Design review of the part shown in the three views and the two pictorial views. Dimensions are in mm from the part's minimum x, y and z. A direction names the side the tool comes from. Give positions to 0.01 mm unless a question says otherwise; leave off trailing zeros. Loops run counter-clockwise (first coordinate to the right, second up) from the corner with the lowest first, then second, coordinate; pieces in that order, holes last. Notation, with made-up numbers: (20.5, -34) - (41.5, -34) arc R36 ccw to (41.5, 5) - close; hole circle Ø7 at (0.5, 81). An arc over 180 degrees is marked (long way). Use CSV: the item, a comma, the result in double quotes. Start each with the question number.
1. Wall thickness on line 1 (Y direction, x = 27, z = 18); line 2 (Y direction, x = 7, z = 19); line 3 (Z direction, x = 19.5, y = 10): over which ranges is each line inside the solid? List them lowest first.
2. For pin 1 (2 mm diameter, centred on y = 30.5, z = 16, fed in from +X); pin 2 (19 mm diameter, centred on x = 10, z = 15.5, fed in from -Y); pin 3 (3 mm diameter, centred on x = 19, y = 26.5, fed in from +Z), all flat-tipped, find the tip position at first contact; note any pin that passes through.
3. Take a section at D-D on z = 19. Give the boundary of the cut face in (x, y), plus the area to 3 significant figures.
4. For the marked faces 1, 2 and 3, list the 3-axis set-ups (+Z, -Z, +X, -X, +Y, -Y) from which the entire face can be reached by the end or side of a thin tool; tool diameter is ignored.
5. Take a section at A-A on x = 19. Give the boundary of the cut face in (y, z).
6. Mouldability with a two-part tool opening along Y and no side actions: class the marked faces 4, 5, 6 and 7 as pulls with the +Y half, pulls with the -Y half, needs draft (parallel to the pull), parting line crosses it, or undercut.
7. Take a section at B-B on z = 6. Give the boundary of the cut face in (x, y), plus the area to 3 significant figures.
8. Take a section at C-C on x = 6. Give the boundary of the cut face in (y, z), plus the area to 3 significant figures.
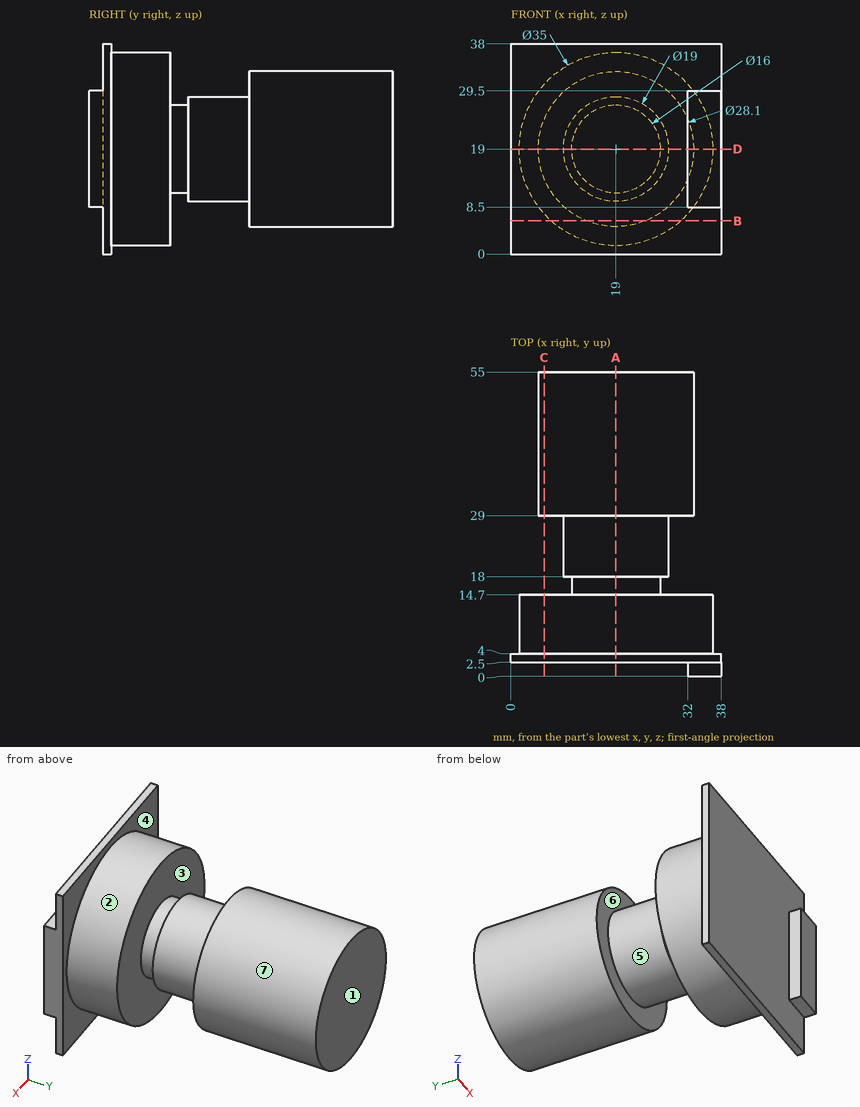
Check result:
1,line 1,"y = 2.5 to 14.7, 18 to 55"
1,line 2,"y = 2.5 to 14.7, 29 to 55"
1,line 3,"z = 1.51 to 36.49"
2,pin 1,"stops at x = 32.91"
2,pin 2,"stops at y = 2.5"
2,pin 3,"stops at z = 28.5"
3,outline,"(0, 2.5) - (32, 2.5) - (32, 0) - (38, 0) - (38, 4) - (36.5, 4) - (36.5, 14.7) - (27, 14.7) - (27, 18) - (28.5, 18) - (28.5, 29) - (33.05, 29) - (33.05, 55) - (4.95, 55) - (4.95, 29) - (9.5, 29) - (9.5, 18) - (11, 18) - (11, 14.7) - (1.5, 14.7) - (1.5, 4) - (0, 4) - close"
3,area,"1,440 mm²"
4,face 1,"+Z, -Z, +X, -X, +Y"
4,face 2,"+Y"
4,face 3,"none"
5,outline,"(2.5, 0) - (4, 0) - (4, 1.5) - (14.7, 1.5) - (14.7, 11) - (18, 11) - (18, 9.5) - (29, 9.5) - (29, 4.95) - (55, 4.95) - (55, 33.05) - (29, 33.05) - (29, 28.5) - (18, 28.5) - (18, 27) - (14.7, 27) - (14.7, 36.5) - (4, 36.5) - (4, 38) - (2.5, 38) - close"
6,face 4,"pulls with the +Y half"
6,face 5,"undercut"
6,face 6,"undercut"
6,face 7,"needs draft"
7,outline,"(0, 2.5) - (38, 2.5) - (38, 4) - (30.72, 4) - (30.72, 14.7) - (7.28, 14.7) - (7.28, 4) - (0, 4) - close; (13.67, 29) - (24.33, 29) - (24.33, 55) - (13.67, 55) - close"
7,area,"585 mm²"
8,outline,"(2.5, 0) - (4, 0) - (4, 7.28) - (14.7, 7.28) - (14.7, 30.72) - (4, 30.72) - (4, 38) - (2.5, 38) - close; (29, 13.67) - (55, 13.67) - (55, 24.33) - (29, 24.33) - close"
8,area,"585 mm²"
